Source: CAD feature listing. Evaluate the final solid. Frame: model axes, mm. Face numbers are marked on the shaded views. A direction names the side the tool comes from. Give positions to 0.01 mm unless a question says otherwise; leave off trailing zeros. Order: outer loops, then holes, each group sorted by start corner. A loop starts at its lowest first (then second) coordinate and runs counter-clockwise, first axis right, second up.
from build123d import *

# Parameters (mm, degrees)
F0_W     = 30
F0_H     = 7.45
F0_W_2   = 6
F0_W_3   = 4.75
F0_H_2   = 12
F0_W_4   = 0.6859594434
F0_W_5   = 0.5640405566
F0_W_6   = 34
F1_DEPTH = 3
F2_DEPTH = 5.5
F3_W     = 5
F3_H     = 2
F4_DEPTH = 25
F6_D     = 1
F7_W     = 10
F7_H     = 2
F8_DEPTH = 25


with BuildPart() as f1:
    # F0 (on Top) → F1 (new body)
    with BuildSketch(Plane.XY):
        with Locations((40, 13.525)):
            Rectangle(F0_W, F0_H)
        with Locations((40, -13.525)):
            Rectangle(F0_W, F0_H)
        with Locations((22, -13.525)):
            Rectangle(F0_W_2, F0_H)
        Polygon((19.6859594434, -6), (19, -6), (19, -9.8), (25, -9.8), (25, -6), (24.4359594434, -6), align=None)
        with Locations((22.0609594434, 0)):
            Rectangle(F0_W_3, F0_H_2)
        with Locations((19.3429797217, 0)):
            Rectangle(F0_W_4, F0_H_2)
        with Locations((24.7179797217, 0)):
            Rectangle(F0_W_5, F0_H_2)
        Polygon((25, 9.8), (19, 9.8), (19, 6), (19.6859594434, 6), (24.4359594434, 6), (25, 6), align=None)
        with Locations((22, 13.525)):
            Rectangle(F0_W_2, F0_H)
        with Locations((2, 13.525)):
            Rectangle(F0_W_6, F0_H)
        with Locations((2, -13.525)):
            Rectangle(F0_W_6, F0_H)
        Polygon((-15, -6.8), (-25, -6.8), (-25, -17.25), (-15, -17.25), (-15, -9.8), align=None)
        Polygon((-15, 17.25), (-25, 17.25), (-25, 6.8), (-15, 6.8), (-15, 9.8), align=None)
    extrude(amount=F1_DEPTH)

    # F0 (on Top) → F2 (join)
    with BuildSketch(Plane.XY):
        with Locations((22.0609594434, 0)):
            Rectangle(F0_W_3, F0_H_2)
    extrude(amount=-F2_DEPTH)

    # F3 (on face) → F4 (cut)
    with BuildSketch(Plane.XY.offset(3)):
        with Locations((-22.5, 12.025)):
            Rectangle(F3_W, F3_H)
        with Locations((-22.5, -12.025)):
            Rectangle(F3_W, F3_H)
    extrude(amount=-F4_DEPTH, mode=Mode.SUBTRACT)

    # F6 (through all)
    with Locations(Plane.XZ.offset(17.25)):
        with Locations((-21.5, 1.5), (51.5, 1.5)):
            Hole(F6_D / 2)

    # F7 (on face) → F8 (cut)
    with BuildSketch(Plane.XY.offset(3)):
        with Locations((55, -13.525)):
            Rectangle(F7_W, F7_H)
        with Locations((55, 13.525)):
            Rectangle(F7_W, F7_H)
    extrude(amount=-F8_DEPTH, mode=Mode.SUBTRACT)


solid = f1.part
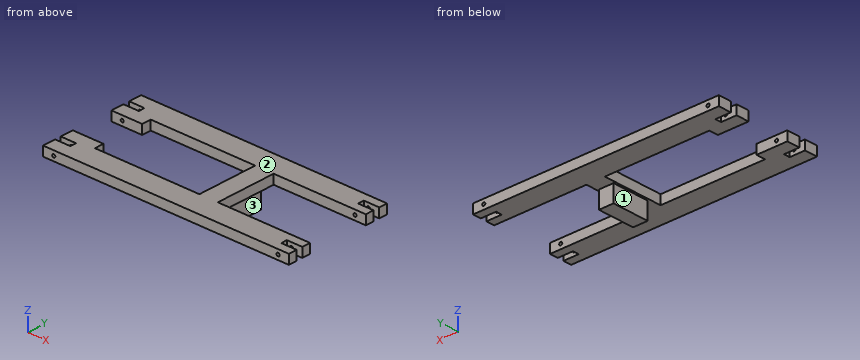
1) Section query B-B on y = -4. Output: boundary loops of the cut face in (x, z).
Checks:
outline: (19, 0) - (19.69, 0) - (19.69, -5.5) - (24.44, -5.5) - (24.44, 0) - (25, 0) - (25, 3) - (19, 3) - close
2) Section query C-C on z = -1.5. Output: boundary loops of the cut face in (x, y), and give its area (3 significant figures).
Checks:
outline: (19.69, -6) - (24.44, -6) - (24.44, 6) - (19.69, 6) - close
area: 57.0 mm2
3) Section query A-A on x = 29.5. Output: boundary loops of the cut face in (y, z).
Checks:
outline: (-17.25, 0) - (-9.8, 0) - (-9.8, 3) - (-17.25, 3) - close; (9.8, 0) - (17.25, 0) - (17.25, 3) - (9.8, 3) - close
4) Ray query, L1, parallel to Y at x = 37, z = 2.5; L2, parallel to Z at x = 51.5, y = 15.1; L3, parallel to Y at x = -18, z = 2. Return the intervals inside material, ascending.
Checks:
L1: y = -17.25 to -9.8, 9.8 to 17.25
L2: z = 0 to 1, 2 to 3
L3: y = -17.25 to -6.8, 6.8 to 17.25
5) First-contact query: pin 1 Ø4 at (x, z) = (21.5, -2.5) entering from +Y; pin 2 Ø3.5 at (y, z) = (-8, 1) entering from +X; pin 3 Ø0.9 at (y, z) = (-1.5, 1.5) entering from -X. Flat tips, straight axial feed; report the tip coordinate or a pass-through.
Checks:
pin 1: stops at y = 6
pin 2: stops at x = 25
pin 3: stops at x = 19
6) Reachability of the marked faces 1, 2 and 3 from +Z, -Z, +X, -X, +Y, -Y: full face, straight path, thin tool, end or side. Return the list, or none.
Checks:
face 1: -Z, -X, +Y, -Y
face 2: +Z, +X, -X, +Y, -Y
face 3: -Z, +X, +Y, -Y
